```python
from build123d import *

# Parameters (mm, degrees)
SKETCH1_W           = 228.346
SKETCH1_H           = 177.8
BOSS_EXTRUDE1_DEPTH = 5.842
FILLET1_R           = 63.5
FILLET2_R           = 63.5
FILLET3_R           = 63.5
SKETCH2_W           = 8.466666667
SKETCH2_H           = 5.842
CUT_EXTRUDE1_DEPTH  = 145.819932651


with BuildPart() as part:
    # Sketch1 → Boss-Extrude1 (new body)
    with BuildSketch(Plane.XY):
        Rectangle(SKETCH1_W, SKETCH1_H)
    extrude(amount=BOSS_EXTRUDE1_DEPTH)

    # Fillet1
    fillet1_edges = [part.edges().sort_by_distance(p)[0] for p in [
        (-114.173, 88.9, 2.921),
    ]]
    fillet(fillet1_edges, radius=FILLET1_R)

    # Fillet2
    fillet2_edges = [part.edges().sort_by_distance(p)[0] for p in [
        (-114.173, -88.9, 2.921),
    ]]
    fillet(fillet2_edges, radius=FILLET2_R)

    # Fillet3
    fillet3_edges = [part.edges().sort_by_distance(p)[0] for p in [
        (114.173, 88.9, 2.921),
        (114.173, -88.9, 2.921),
    ]]
    fillet(fillet3_edges, radius=FILLET3_R)

    # Sketch2 → Cut-Extrude1 (cut, through all)
    with BuildSketch(Plane.XY.offset(5.842)):
        with Locations((4.360333334, -28.321)):
            Rectangle(SKETCH2_W, SKETCH2_H)
        with Locations((21.293666667, -28.321)):
            Rectangle(SKETCH2_W, SKETCH2_H)
        with Locations((4.360333334, 28.321)):
            Rectangle(SKETCH2_W, SKETCH2_H)
        with Locations((21.293666667, 28.321)):
            Rectangle(SKETCH2_W, SKETCH2_H)
        with Locations((-96.731666667, -28.321)):
            Rectangle(SKETCH2_W, SKETCH2_H)
        with Locations((-79.798333334, -28.321)):
            Rectangle(SKETCH2_W, SKETCH2_H)
        with Locations((-96.731666667, 28.321)):
            Rectangle(SKETCH2_W, SKETCH2_H)
        with Locations((-79.798333334, 28.321)):
            Rectangle(SKETCH2_W, SKETCH2_H)
    extrude(amount=-CUT_EXTRUDE1_DEPTH, mode=Mode.SUBTRACT)


solid = part.part
```
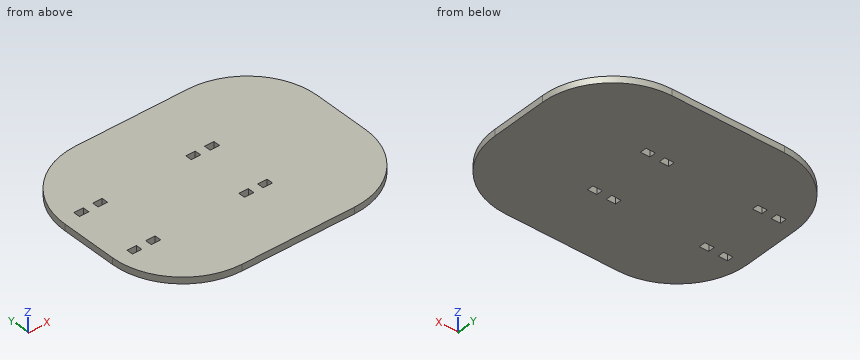
CAD build for the part. Positions are in the model's coordinates, mm. Round coordinates to 2 decimals unless told otherwise and drop trailing zeros. Order: outer loops, then holes, each group sorted by start corner. A loop starts at its lowest first (then second) coordinate and runs counter-clockwise, first axis right, second up. Notation, with made-up numbers: (0, 14) -> (4, 14) arc R20 ccw to (4, 28) -> close; hole circle Ø7 at (-37.75, 29.25). An arc over 180 degrees is marked (long way). One line per question, with ' | ' between items.
Q1. Drop flat-ended pins along their axis: pin 1 (1.8 mm diameter, centred on y = -27, z = 3.5, fed in from +X); pin 2 (3 mm diameter, centred on y = -28, z = 4, fed in from -X); pin 3 (1.8 mm diameter, centred on y = 28, z = 3, fed in from -X). Give the stop position or say it passes through.
Completed:
pin 1: stops at x = 114.17 | pin 2: stops at x = -114.16 | pin 3: stops at x = -114.15
Q2. Slice it at B-B (z = 2.8). Give the number of separate pieces and of enclosed holes in the cut face, then the cut area to 3 significant figures.
Completed:
separate pieces: 1 | enclosed holes: 8 | area: 36,700 mm^2
Q3. Slice it at D-D (y = -69.5). Write the cut outline in (x, z), then the cut area to 3 significant figures.
Completed:
outline: (-96.36, 0) -> (96.36, 0) -> (96.36, 5.84) -> (-96.36, 5.84) -> close | area: 1,130 mm^2
Q4. Probe probe 1 along X at (y, z) = (-40.5, 5.5); probe 2 along Y at (x, z) = (105.5, 4.9); probe 3 along Y at (x, z) = (-53, 1.05). List the from-to ranges inside material, lowest first.
Completed:
probe 1: x = -112.35 to 112.35 | probe 2: y = -57.44 to 57.44 | probe 3: y = -88.86 to 88.86
Q5. Slice it at A-A (x = 20.5). Write the cut outline in (y, z).
Completed:
outline: (-88.9, 0) -> (-31.24, 0) -> (-31.24, 5.84) -> (-88.9, 5.84) -> close; (-25.4, 0) -> (25.4, 0) -> (25.4, 5.84) -> (-25.4, 5.84) -> close; (31.24, 0) -> (88.9, 0) -> (88.9, 5.84) -> (31.24, 5.84) -> close
Q6. Slice it at C-C (x = -95.5). Write the cut outline in (y, z).
Completed:
outline: (-70.38, 0) -> (-31.24, 0) -> (-31.24, 5.84) -> (-70.38, 5.84) -> close; (-25.4, 0) -> (25.4, 0) -> (25.4, 5.84) -> (-25.4, 5.84) -> close; (31.24, 0) -> (70.38, 0) -> (70.38, 5.84) -> (31.24, 5.84) -> close
